Model file for the job. Use its own axes, mm. Face numbers are marked on the shaded views. Coordinates: 2 decimals unless noted, no trailing zeros. Write each loop counter-clockwise with the first axis right and the second up, starting at its lowest first coordinate (ties: lowest second). Pieces come first, ordered by that corner, then holes.
Q1. Pull direction Y, two halves, no side cores. Call the marked faces 1, 2 and 3: released by +Y, released by -Y, zero draft, split by the parting line, or undercut.
Q2. Band-saw the part on B-B, the plane z = 5.75. Write the cut outline in (x, y).
Q3. Band-saw the part on A-A, the plane z = 8. Write the cut outline in (x, y).
Q4. Drill centre lines: probe 1 along X at (y, z) = (0.75, 7); probe 2 along Z at (x, y) = (-0.5, 0). Where is each one in solid material? Low to high.
Q5. Pin check, flat tips, straight feed: P1, Ø0.9, axis at y = -1.5, z = 9, coming from the +X side; P2, Ø0.9, axis at x = 1.5, z = 10.5, coming from the +Y side; P3, Ø2.5, axis at x = 0.5, y = 0.5, coming from the +Z side; P4, Ø1.2, axis at x = -2, z = 10, coming from the -Y side. Stop position of each tip, or through.
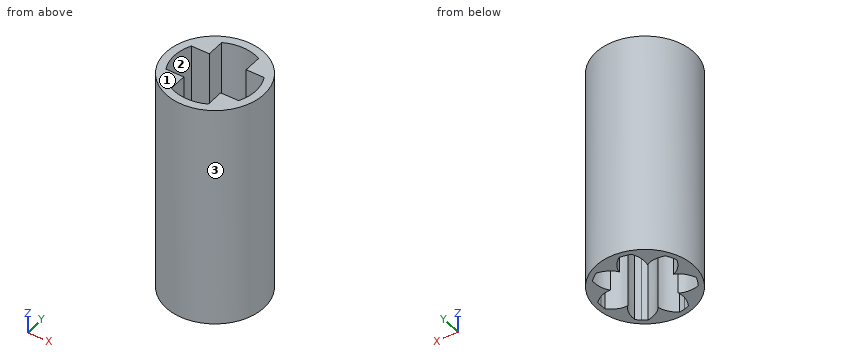
from build123d import *

# Parameters (mm, degrees)
SKETCH_1_R               = 3
SKETCH_1_R_2             = 1.5625
EXTRUDE_1_DEPTH          = 5
CUT_EXTRUDE_2_DEPTH      = 7.557438524
PATTERN_CIRCULAR_1_COUNT = 7
SKETCH_2_R               = 3
EXTRUDE_2_DEPTH          = 8.8
CUT_EXTRUDE_START        = 8.8
CUT_EXTRUDE_3_DEPTH      = 7.8


with BuildPart() as part:
    # 草图1 → 凸台-拉伸1 (new body)
    with BuildSketch(Plane.XY):
        Circle(SKETCH_1_R)
        Circle(SKETCH_1_R_2, mode=Mode.SUBTRACT)
    extrude(amount=EXTRUDE_1_DEPTH)

    # 草图1<3> → 切除-拉伸2 (cut, through all)
    with BuildSketch(Plane.XY):
        with BuildLine():
            Line((1.473941588, 0.729213103), (1.40047846, 0.692868192))
            ThreePointArc((1.40047846, 0.692868192), (1.521455528, 0.355779887), (1.5625, 0))
            ThreePointArc((1.5625, 0), (1.521455528, -0.355779887), (1.40047846, -0.692868192))
            Line((1.40047846, -0.692868192), (1.473941588, -0.729213103))
            add(Edge.make_bspline(
                [(1.473941588, -0.729213103), (1.485175683, -0.734771023), (1.517731995, -0.74785023), (1.58325759, -0.763025647), (1.69185053, -0.772739945), (1.833066262, -0.76334643), (2.010800821, -0.725727848), (2.210262557, -0.650798613), (2.403274907, -0.54458002), (2.544769721, -0.44101945), (2.63009006, -0.368231772), (2.666526001, -0.335104965)],
                knots=[0, 0, 0, 0, 0, 0.005604068, 0.015718248, 0.029959916, 0.048733667, 0.068727063, 0.096888892, 0.125050566, 0.147116643, 0.147116643, 0.147116643, 0.147116643, 0.147116643], degree=4))
            ThreePointArc((2.666526001, -0.335104965), (2.682251375, -0.167880349), (2.6875, 0))
            ThreePointArc((2.6875, 0), (2.682251375, 0.167880349), (2.666526001, 0.335104965))
            add(Edge.make_bspline(
                [(1.473941588, 0.729213103), (1.485175683, 0.734771023), (1.517731995, 0.74785023), (1.58325759, 0.763025647), (1.69185053, 0.772739945), (1.833066262, 0.76334643), (2.010800821, 0.725727848), (2.210262557, 0.650798613), (2.403274907, 0.54458002), (2.544769721, 0.44101945), (2.63009006, 0.368231772), (2.666526001, 0.335104965)],
                knots=[0, 0, 0, 0, 0, 0.005604068, 0.015718248, 0.029959916, 0.048733667, 0.068727063, 0.096888892, 0.125050566, 0.147116643, 0.147116643, 0.147116643, 0.147116643, 0.147116643], degree=4))
        make_face()
    cut_extrude_2 = extrude(amount=CUT_EXTRUDE_2_DEPTH, mode=Mode.SUBTRACT)

    # 阵列(圆周)1: 切除-拉伸2 ×7 about axis
    pattern_circular_1_axis = Axis((0, 0, 5), (0, 0, 1))
    for i in range(1, PATTERN_CIRCULAR_1_COUNT):
        add(cut_extrude_2.rotate(pattern_circular_1_axis, i * 360 / PATTERN_CIRCULAR_1_COUNT), mode=Mode.SUBTRACT)

    # 草图2 → 凸台-拉伸2 (add)
    with BuildSketch(Plane.XY.offset(5)):
        Circle(SKETCH_2_R)
    extrude(amount=EXTRUDE_2_DEPTH)

    # 草图2<4> → 切除-拉伸3 (cut)
    with BuildSketch(Plane.XY.offset(5).offset(CUT_EXTRUDE_START)):
        with BuildLine():
            ThreePointArc((1.130029762, 2.230029762), (0, 2.5), (-1.130029762, 2.230029762))
            Line((-1.130029762, 2.230029762), (-1.130029762, 1.130029762))
            Line((-1.130029762, 1.130029762), (-2.230029762, 1.130029762))
            ThreePointArc((-2.230029762, 1.130029762), (-2.5, 0), (-2.230029762, -1.130029762))
            Line((-2.230029762, -1.130029762), (-1.130029762, -1.130029762))
            Line((-1.130029762, -1.130029762), (-1.130029762, -2.230029762))
            ThreePointArc((-1.130029762, -2.230029762), (0, -2.5), (1.130029762, -2.230029762))
            Line((1.130029762, -2.230029762), (1.130029762, -1.130029762))
            Line((1.130029762, -1.130029762), (2.230029762, -1.130029762))
            ThreePointArc((2.230029762, -1.130029762), (2.5, 0), (2.230029762, 1.130029762))
            Line((2.230029762, 1.130029762), (1.130029762, 1.130029762))
            Line((1.130029762, 1.130029762), (1.130029762, 2.230029762))
        make_face()
    extrude(amount=-CUT_EXTRUDE_3_DEPTH, mode=Mode.SUBTRACT)


solid = part.part
Answer sheet:
1. face 1: zero draft
1. face 2: undercut
1. face 3: split by the parting line
2. outline: circle Ø6 at (0, 0)
3. outline: circle Ø6 at (0, 0); hole (-2.23, -1.13) - (-1.13, -1.13) - (-1.13, -2.23) arc R2.5 ccw to (1.13, -2.23) - (1.13, -1.13) - (2.23, -1.13) arc R2.5 ccw to (2.23, 1.13) - (1.13, 1.13) - (1.13, 2.23) arc R2.5 ccw to (-1.13, 2.23) - (-1.13, 1.13) - (-2.23, 1.13) arc R2.5 ccw to start
4. probe 1: x = -2.9 to -2.38, 2.38 to 2.9
4. probe 2: z = 5 to 6
5. P1: stops at x = 2.81
5. P2: stops at y = 2.81
5. P3: stops at z = 13.8
5. P4: stops at y = -2.65
